from build123d import *

# Parameters (mm, degrees)
EXTRUDE_1_DEPTH             = 10
HOLE_WIZARD_M43_D           = 4.5
HOLE_WIZARD_M43_CBORE_D     = 8
HOLE_WIZARD_M43_CBORE_DEPTH = 4
FILLET_4_R                  = 2
FILLET_2_R                  = 3


with BuildPart() as part:
    # Эскиз1 → Бобышка-Вытянуть1 (new body)
    with BuildSketch(Plane.XY):
        with BuildLine():
            Line((-31.75, 5), (-4.101162824, 13.438116069))
            ThreePointArc((-4.101162824, 13.438116069), (0, 14.05), (4.101162824, 13.438116069))
            Line((4.101162824, 13.438116069), (31.75, 5))
            Line((31.75, 5), (31.75, 0))
            Line((31.75, 0), (11.05, 0))
            ThreePointArc((11.05, 0), (0, 11.05), (-11.05, 0))
            Line((-11.05, 0), (-31.75, 0))
            Line((-31.75, 0), (-31.75, 5))
        make_face()
    extrude(amount=EXTRUDE_1_DEPTH)

    # Эскиз5 → Цековка для винта с внутренним шестигранником M42 (revolve, cut)
    with BuildSketch(Plane(origin=(-26.75, 7, 5), x_dir=(0, 0, -1), z_dir=(1, 0, 0))):
        Polygon((0, 0), (0, 7.05), (2.25, 7.05), (2.25, 4), (4, 4), (4, 0), align=None)
    revolve(axis=Axis((-26.75, 0.65, 5), (0, 1, 0)), mode=Mode.SUBTRACT)

    # Цековка для винта с внутренним шестигранником M43 (through all)
    with Locations(Plane(origin=(0, 7, 0), x_dir=(1, 0, 0), z_dir=(0, 1, 0))):
        with Locations((-26.75, -5)):
            CounterBoreHole(HOLE_WIZARD_M43_D / 2, HOLE_WIZARD_M43_CBORE_D / 2, HOLE_WIZARD_M43_CBORE_DEPTH)

    # Эскиз10 → Цековка для винта с внутренним шестигранником M44 (revolve, cut)
    with BuildSketch(Plane(origin=(26.75, 7, 5), x_dir=(0, 0, 1), z_dir=(1, 0, 0))):
        Polygon((0, 0), (0, 7), (2.25, 7), (2.25, 4), (4, 4), (4, 0), align=None)
    revolve(axis=Axis((26.75, 13.35, 5), (0, -1, 0)), mode=Mode.SUBTRACT)

    # Эскиз12 → Цековка для винта с внутренним шестигранником M45 (revolve, cut)
    with BuildSketch(Plane(origin=(26.75, 7, 5), x_dir=(0, 0, -1), z_dir=(1, 0, 0))):
        Polygon((0, 0), (0, 7.05), (2.25, 7.05), (2.25, 4), (4, 4), (4, 0), align=None)
    revolve(axis=Axis((26.75, 0.65, 5), (0, 1, 0)), mode=Mode.SUBTRACT)

    # Скругление4
    fillet_4_edges = [part.edges().sort_by_distance(p)[0] for p in [
        (-11.05, 0, 5),
        (11.05, 0, 5),
    ]]
    fillet(fillet_4_edges, radius=FILLET_4_R)

    # Скругление2
    # the kernel refuses this fillet: 3 mm, written as the material it takes off along each edge
    with BuildSketch(Plane(origin=(-31.75, 5, -5.552584785), x_dir=(0, -1, 0), z_dir=(0, 0, 1)), Plane(origin=(31.75, 5, -5.552584785), x_dir=(-0.95644954230243, 0.2918977098736336, 0), z_dir=(0, 0, 1))) as fillet_2_piece_1:
        with BuildLine():
            CenterArc((FILLET_2_R * 0.740344637964, FILLET_2_R), FILLET_2_R, 196.971603354, 73.028396646)
            Line((-FILLET_2_R * 0.216104904339, FILLET_2_R * 0.708102290126), (0, 0))
            Line((0, 0), (FILLET_2_R * 0.740344637964, 0))
        make_face()
    extrude(amount=21.105169569, mode=Mode.SUBTRACT)


solid = part.part
Model file for the job. Use its own axes, mm. A direction names the side the tool comes from. Round coordinates to 2 decimals unless told otherwise and drop trailing zeros. Order: outer loops, then holes, each group sorted by start corner. A loop starts at its lowest first (then second) coordinate and runs counter-clockwise, first axis right, second up.
(1) Drill centre lines: line 1 (Z direction, x = 26.75, y = 5.4); line 2 (Z direction, x = -26.75, y = 0.8); line 3 (X direction, y = 3.9, z = 5). Where is each one in solid material? Low to high.
(2) Pin check, flat tips, straight feed: pin 1 (2.5 mm diameter, centred on x = -26.75, z = 5, fed in from +Y); pin 2 (2.5 mm diameter, centred on x = 25.5, z = 3.5, fed in from +Y); pin 3 (1 mm diameter, centred on x = 9.5, z = 5.5, fed in from +Y); pin 4 (1.5 mm diameter, centred on x = 19, z = 2.5, fed in from +Y). Stop position of each tip, or through.
(3) Band-saw the part on B-B (z = 6.5). List the corners of the cut face in (x, y).
(4) 3-axis set-ups, long thin cutter, end or side, ignore diameter. For faces 4 (the face through (-14.206, 10.354, 4.93)), 5 (the face through (28.5, 3, 3.3)), 6 (the face through (11.61, 0.47, 5.07)): which of +Z, -Z, +X, -X, +Y, -Y reach the whole face in a straight line?
(5) Pull direction X, two halves, no side cores. Call faces 1 (the face through (-31.376, 4.229, 4.93)), 2 (the face through (31.18, 4.54, 4.93)), 3 (the face through (-28.896, 1.479, 4.324)): released by +X, released by -X, zero draft, split by the parting line, or undercut.
(6) Band-saw the part on A-A (y = 4.5). List the corners of the cut face in (x, z).
(7) Band-saw the part on D-D (x = -23.5). List the corners of the cut face in (y, z), then the cut area to 3 significant figures.
(8) Band-saw the part on C-C (x = 26.75). List the corners of the cut face in (y, z).
Verdict:
1. line 1: z = 0 to 1, 9 to 10
1. line 2: z = 0 to 2.75, 7.25 to 10
1. line 3: x = -31.53 to -30.75, -22.75 to -10.34, 10.34 to 22.75, 30.75 to 31.53
2. pin 1: passes through
2. pin 2: stops at y = 3
2. pin 3: stops at y = 11.94
2. pin 4: stops at y = 9.12
3. outline: (-31.75, 0) - (-28.43, 0) - (-28.43, 3) - (-30.46, 3) - (-30.46, 5.25) arc R3 ccw to (-31.75, 2.78) - close; (-25.07, 0) - (-12.9, 0) arc R2 ccw to (-10.92, 1.69) arc R11.05 cw to (10.92, 1.69) arc R2 ccw to (12.9, 0) - (25.07, 0) - (25.07, 3) - (23.04, 3) - (23.04, 7.66) - (4.1, 13.44) arc R14.05 ccw to (-4.1, 13.44) - (-23.04, 7.66) - (-23.04, 3) - (-25.07, 3) - close; (28.43, 0) - (31.75, 0) - (31.75, 2.78) arc R3 ccw to (30.46, 5.25) - (30.46, 3) - (28.43, 3) - close
4. face 4: +Z, -Z, -X, +Y
4. face 5: +Y
4. face 6: +Z, -Z, -Y
5. face 1: released by -X
5. face 2: released by +X
5. face 3: undercut
6. outline: (-31.21, 0) - (-10.09, 0) - (-10.09, 10) - (-31.21, 10) - close; (10.09, 0) - (31.21, 0) - (31.21, 10) - (10.09, 10) - close; hole circle Ø8 at (-26.75, 5); hole circle Ø8 at (26.75, 5)
7. outline: (0, 0) - (7.52, 0) - (7.52, 2.67) - (3, 2.67) - (3, 7.33) - (7.52, 7.33) - (7.52, 10) - (0, 10) - close
7. area: 54.1 mm2
8. outline: (0, 0) - (6.53, 0) - (6.53, 1) - (3, 1) - (3, 2.75) - (0, 2.75) - close; (0, 7.25) - (3, 7.25) - (3, 9) - (6.53, 9) - (6.53, 10) - (0, 10) - close
